```python
from build123d import *

# Parameters (mm, degrees)
SKETCH2_R           = 17.5
SKETCH2_R_2         = 2.25
BOSS_EXTRUDE1_DEPTH = 5
SKETCH3_R           = 10
BOSS_EXTRUDE2_DEPTH = 15
SKETCH4_R           = 2.5
CUT_EXTRUDE1_DEPTH  = 32.819805153


with BuildPart() as part:
    # Sketch2 → Boss-Extrude1 (new body)
    with BuildSketch(Plane(origin=(0, 0, 0), x_dir=(1, 0, 0), z_dir=(0, 1, 0))):
        with Locations(Location((0, 0, 0), (0, 0, 270))):
            Circle(SKETCH2_R)
        with Locations(Location((0, 13.75, 0), (0, 0, 270))):
            Circle(SKETCH2_R_2, mode=Mode.SUBTRACT)
        with Locations(Location((11.907849302, 6.875, 0), (0, 0, 270))):
            Circle(SKETCH2_R_2, mode=Mode.SUBTRACT)
        with Locations(Location((11.907849302, -6.875, 0), (0, 0, 270))):
            Circle(SKETCH2_R_2, mode=Mode.SUBTRACT)
        with Locations(Location((0, -13.75, 0), (0, 0, 270))):
            Circle(SKETCH2_R_2, mode=Mode.SUBTRACT)
        with Locations(Location((-11.907849302, -6.875, 0), (0, 0, 270))):
            Circle(SKETCH2_R_2, mode=Mode.SUBTRACT)
        with Locations(Location((-11.907849302, 6.875, 0), (0, 0, 270))):
            Circle(SKETCH2_R_2, mode=Mode.SUBTRACT)
    extrude(amount=BOSS_EXTRUDE1_DEPTH)

    # Sketch3 → Boss-Extrude2 (add)
    with BuildSketch(Plane(origin=(0, 5, 0), x_dir=(1, 0, 0), z_dir=(0, 1, 0))):
        with Locations(Location((0, 0, 0), (0, 0, 270))):
            Circle(SKETCH3_R)
    extrude(amount=BOSS_EXTRUDE2_DEPTH)

    # Sketch4 → Cut-Extrude1 (cut, through all)
    with BuildSketch(Plane(origin=(0, 20, 0), x_dir=(1, 0, 0), z_dir=(0, 1, 0))):
        with Locations(Location((0, 0, 0), (0, 0, 270))):
            Circle(SKETCH4_R)
    extrude(amount=-CUT_EXTRUDE1_DEPTH, mode=Mode.SUBTRACT)


solid = part.part
```
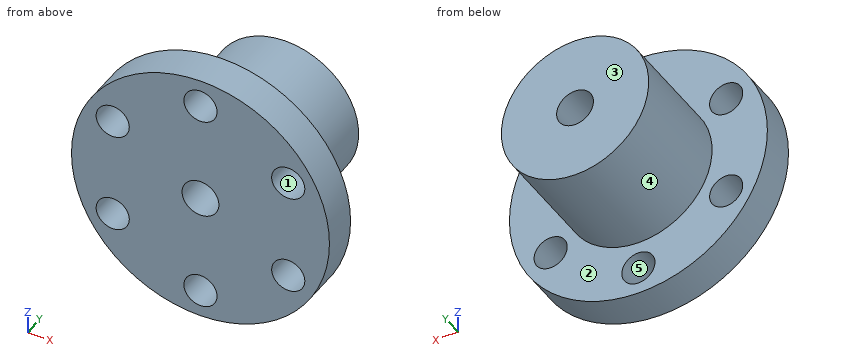
Verification items for the finished model (mm, model axes). Face numbers are marked on the shaded views. A direction names the side the tool comes from. Give positions to 0.01 mm unless a question says otherwise; leave off trailing zeros. Order: outer loops, then holes, each group sorted by start corner. A loop starts at its lowest first (then second) coordinate and runs counter-clockwise, first axis right, second up. Notation, with made-up numbers: (-28.5, 47.5) -> (25.5, 47.5) arc R18 ccw to (25.5, 68.5) -> close; hole circle Ø6 at (-32, -30). An arc over 180 degrees is marked (long way). One line per item, written item: value.
(1) Sectioned sample at C-C on z = 6. Record the cut outline in (x, y).
Final values:
outline: (-16.44, 0) -> (-13.98, 0) -> (-13.98, 5) -> (-16.44, 5) -> close; (-9.83, 0) -> (9.83, 0) -> (9.83, 5) -> (8, 5) -> (8, 20) -> (-8, 20) -> (-8, 5) -> (-9.83, 5) -> close; (13.98, 0) -> (16.44, 0) -> (16.44, 5) -> (13.98, 5) -> close
(2) Tool access check on the marked faces 1 and 2. Record the directions out of +Z, -Z, +X, -X, +Y, -Y that give a thin tool (end or side, any length) a straight path to the whole face; none if there is none.
Final values:
face 1: +Y, -Y
face 2: +Y
(3) Sectioned sample at D-D on y = 3.5. Record the cut outline in (x, z) (3 decimals).
Final values:
outline: circle Ø35 at (0, 0); hole circle Ø4.5 at (-11.908, -6.875); hole circle Ø4.5 at (-11.908, 6.875); hole circle Ø5 at (0, 0); hole circle Ø4.5 at (0, -13.75); hole circle Ø4.5 at (0, 13.75); hole circle Ø4.5 at (11.908, -6.875); hole circle Ø4.5 at (11.908, 6.875)
(4) Sectioned sample at A-A on x = 0. Record the cut outline in (y, z).
Final values:
outline: (0, -17.5) -> (5, -17.5) -> (5, -16) -> (0, -16) -> close; (0, -11.5) -> (5, -11.5) -> (5, -10) -> (20, -10) -> (20, -2.5) -> (0, -2.5) -> close; (0, 2.5) -> (20, 2.5) -> (20, 10) -> (5, 10) -> (5, 11.5) -> (0, 11.5) -> close; (0, 16) -> (5, 16) -> (5, 17.5) -> (0, 17.5) -> close
(5) Gauge pin test, flat ends, axial feed: pin 1 (5 mm diameter, centred on x = 11.91, z = 6.88, fed in from +Y); pin 2 (1 mm diameter, centred on x = 5, y = 6, fed in from +Z); pin 3 (1.5 mm diameter, centred on x = -12.5, y = 4, fed in from -Z); pin 4 (2 mm diameter, centred on x = 11.5, z = 8.5, fed in from -Y). Record the tip position at first contact, or that the pin passes through.
Final values:
pin 1: y = 5
pin 2: z = 8.93
pin 3: z = -12.97
pin 4: y = 0
(6) Sectioned sample at B-B on z = 0. Record the cut outline in (x, y).
Final values:
outline: (-17.5, 0) -> (-2.5, 0) -> (-2.5, 20) -> (-10, 20) -> (-10, 5) -> (-17.5, 5) -> close; (2.5, 0) -> (17.5, 0) -> (17.5, 5) -> (10, 5) -> (10, 20) -> (2.5, 20) -> close
(7) Scan lines: line 1 along Z through (x, y) = (1, 3.75); line 2 along Z through (x, y) = (10.5, 4.5); line 3 along Y through (x, z) = (9, 5). Record each from-to range of solid material in increasing order. Write a range as [from, to].
Final values:
line 1: [-17.47, -15.77], [-11.73, -2.29], [2.29, 11.73], [15.77, 17.47]
line 2: [-14, -8.63], [-5.12, 5.12], [8.63, 14]
line 3: [0, 5]
(8) Draft check along Z on the marked faces 3, 4 and 5. Enter one of: pulls with the +Z half, pulls with the -Z half, needs draft (parallel to the pull), parting line crosses it, or undercut.
Final values:
face 3: needs draft
face 4: parting line crosses it
face 5: undercut
